The model under review builds one solid part; all positions refer to its coordinate system, in mm. A direction names the side the tool comes from. Coordinates: 2 decimals unless noted, no trailing zeros. Order: outer loops, then holes, each group sorted by start corner. A loop starts at its lowest first (then second) coordinate and runs counter-clockwise, first axis right, second up. Notation, with made-up numbers: (79, -14) -> (122, -14) arc R25 ccw to (122, 15) -> close; hole circle Ø11 at (72, -27). An arc over 180 degrees is marked (long way). Put each result on its own line as item: value.
from build123d import *

# Parameters (mm, degrees)
SKETCH_R     = 1.75
PAD_DEPTH    = 24.4
SKETCH001_W  = 10
SKETCH001_H  = 18.4
POCKET_DEPTH = 26.5
SKETCH002_W  = 10
SKETCH002_H  = 24.4
PAD001_DEPTH = 3


with BuildPart() as part:
    # Sketch → Pad (new body)
    with BuildSketch(Plane.YZ):
        with BuildLine():
            Line((-13.75, 5), (10.75, 5))
            ThreePointArc((12.75, 3), (12.164214, 4.414214), (10.75, 5))
            Line((12.75, 3), (12.75, -3))
            ThreePointArc((10.75, -5), (12.164214, -4.414214), (12.75, -3))
            Line((10.75, -5), (-13.75, -5))
            Line((-13.75, -5), (-13.75, 5))
        make_face()
        with Locations((-8.75, 0)):
            Circle(SKETCH_R, mode=Mode.SUBTRACT)
        with Locations((8.75, 0)):
            Circle(SKETCH_R, mode=Mode.SUBTRACT)
    extrude(amount=PAD_DEPTH)

    # Sketch001 → Pocket (cut)
    with BuildSketch(Plane(origin=(0, -13.75, 0), x_dir=(0, 0, -1), z_dir=(0, -1, 0))):
        with Locations((0, 12.2)):
            Rectangle(SKETCH001_W, SKETCH001_H)
    extrude(amount=-POCKET_DEPTH, mode=Mode.SUBTRACT)

    # Sketch002 → Pad001 (new body)
    with BuildSketch(Plane(origin=(0, -13.75, 0), x_dir=(0, 0, -1), z_dir=(0, -1, 0))):
        with Locations((0, 12.2)):
            Rectangle(SKETCH002_W, SKETCH002_H)
    extrude(amount=PAD001_DEPTH)


solid = part.part
Item 1: For line 1 (Y direction, x = 1.65, z = 0); line 2 (X direction, y = 8, z = -3.5); line 3 (Z direction, x = 23.75, y = -8.75), list the stretches that pass through material, from the lowest coordinate up. Write a range as from..to.
Answers below:
line 1: -16.75..-10.5, -7..7, 10.5..12.75
line 2: 0..3, 21.4..24.4
line 3: -5..-1.75, 1.75..5
Item 2: For faces 1 (the flat face through (3, -1, 0)), 2 (the flat face through (0, -2, 0)), list the 3-axis set-ups (+Z, -Z, +X, -X, +Y, -Y) from which the entire face can be reached by the end or side of a thin tool; tool diameter is ignored.
Answers below:
face 1: +Z, -Z, +Y
face 2: +Z, -Z, -X, +Y, -Y
Item 3: For pin 1 Ø4.5 at (y, z) = (-8.75, 0) entering from +X; pin 2 Ø6 at (x, z) = (15.5, -3) entering from +Y; pin 3 Ø2 at (y, z) = (8.75, 0) entering from +X, all flat-tipped, find the tip position at first contact; note any pin that passes through.
Answers below:
pin 1: x = 24.4
pin 2: y = -13.75
pin 3: through
Item 4: Mouldability with a two-part tool opening along Y and no side actions: class faces 3 (the flat face through (12, -13.75, 0)), 4 (the cylindrical face through (1.479, 10.419, 0.526)), 5 (the cylindrical face through (1.479, -7.081, 0.526)), 6 (the flat face through (12, -14, -5)) as +Y half, -Y half, draft (parallel to the pull), parting line (faces both ways), or undercut.
Answers below:
face 3: +Y half
face 4: undercut
face 5: undercut
face 6: draft
Item 5: Consider section A-A on z = 0. Write out the cut boundary in (x, y), and give its area (3 significant figures).
Answers below:
outline: (0, -16.75) -> (24.4, -16.75) -> (24.4, -10.5) -> (21.4, -10.5) -> (21.4, -13.75) -> (3, -13.75) -> (3, -10.5) -> (0, -10.5) -> close; (0, -7) -> (3, -7) -> (3, 7) -> (0, 7) -> close; (0, 10.5) -> (3, 10.5) -> (3, 12.75) -> (0, 12.75) -> close; (21.4, -7) -> (24.4, -7) -> (24.4, 7) -> (21.4, 7) -> close; (21.4, 10.5) -> (24.4, 10.5) -> (24.4, 12.75) -> (21.4, 12.75) -> close
area: 190 mm^2
Item 6: Consider section B-B on y = 8.75. Write out the cut boundary in (x, z).
Answers below:
outline: (0, -5) -> (3, -5) -> (3, -1.75) -> (0, -1.75) -> close; (0, 1.75) -> (3, 1.75) -> (3, 5) -> (0, 5) -> close; (21.4, -5) -> (24.4, -5) -> (24.4, -1.75) -> (21.4, -1.75) -> close; (21.4, 1.75) -> (24.4, 1.75) -> (24.4, 5) -> (21.4, 5) -> close
Item 7: Consider section D-D on x = 10.5. Write out the cut boundary in (y, z).
Answers below:
outline: (-16.75, -5) -> (-13.75, -5) -> (-13.75, 5) -> (-16.75, 5) -> close
Item 8: Consider section C-C on y = -5.75. Write out the cut boundary in (x, z).
Answers below:
outline: (0, -5) -> (3, -5) -> (3, 5) -> (0, 5) -> close; (21.4, -5) -> (24.4, -5) -> (24.4, 5) -> (21.4, 5) -> close
